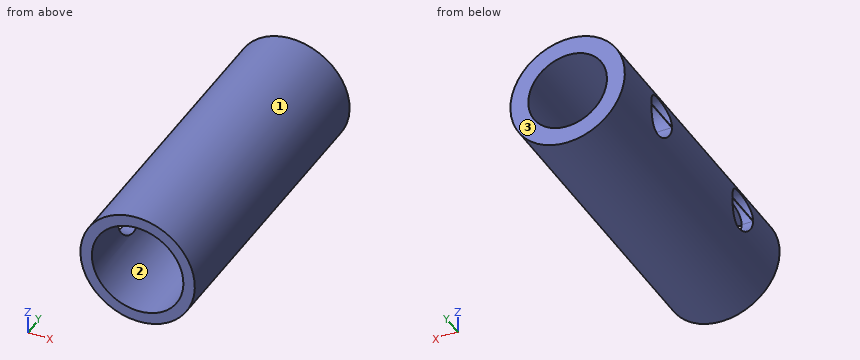
```python
from build123d import *

# Parameters (mm, degrees)
SKETCH1_R           = 4
BOSS_EXTRUDE1_DEPTH = 21
SKETCH2_R           = 3.2
CUT_EXTRUDE1_DEPTH  = 10
SKETCH3_R           = 2.75
CUT_EXTRUDE3_DEPTH  = 10


with BuildPart() as part:
    # Sketch1 → Boss-Extrude1 (new body)
    with BuildSketch(Plane(origin=(0, 0, 0), x_dir=(1, 0, 0), z_dir=(0, 1, 0))):
        with Locations(Location((0, 0, 0), (0, 0, 90))):
            Circle(SKETCH1_R)
    extrude(amount=BOSS_EXTRUDE1_DEPTH)

    # Sketch2 → Cut-Extrude1 (cut)
    with BuildSketch(Plane.XZ):
        with Locations(Location((0, 0, 0), (0, 0, 270))):
            Circle(SKETCH2_R)
    extrude(amount=-CUT_EXTRUDE1_DEPTH, mode=Mode.SUBTRACT)

    # Sketch3 → Cut-Extrude3 (cut)
    with BuildSketch(Plane(origin=(0, 21, 0), x_dir=(1, 0, 0), z_dir=(0, 1, 0))):
        with Locations(Location((0, 0, 0), (0, 0, 270))):
            Circle(SKETCH3_R)
    extrude(amount=-CUT_EXTRUDE3_DEPTH, mode=Mode.SUBTRACT)

    # Cut-Extrude5: read off the stored shape, not the designer's step
    # Cut-Extrude5: loft between two sections, ruled curve by curve
    cut_extrude5_from = [
        Edge.make_three_point_arc((-2.36677924, 14.6, 0), (-2.36677924, 16, 1.4), (-2.36677924, 17.4, 0)),
        Edge.make_three_point_arc((-2.36677924, 17.4, 0), (-2.36677924, 16, -1.4), (-2.36677924, 14.6, 0)),
    ]
    cut_extrude5_to = [
        Edge.make_three_point_arc((-3.999916451, 14.6, 0), (-3.999916451, 16, 1.4), (-3.999916451, 17.4, 0)),
        Edge.make_three_point_arc((-3.999916451, 17.4, 0), (-3.999916451, 16, -1.4), (-3.999916451, 14.6, 0)),
    ]
    cut_extrude5 = Solid(Shell([*[Face.make_surface_from_curves(cut_extrude5_from[k], cut_extrude5_to[k]) for k in range(2)], Face(Wire(cut_extrude5_from)), Face(Wire(cut_extrude5_to))]))
    add(cut_extrude5, mode=Mode.SUBTRACT)

    # Cut-Extrude5 2: loft between two sections, ruled curve by curve
    cut_extrude5_2_from = [
        Edge.make_three_point_arc((-2.877351837, 3.6, 0), (-2.877351837, 5, 1.4), (-2.877351837, 6.4, 0)),
        Edge.make_three_point_arc((-2.877351837, 6.4, 0), (-2.877351837, 5, -1.4), (-2.877351837, 3.6, 0)),
    ]
    cut_extrude5_2_to = [
        Edge.make_three_point_arc((-3.999916451, 3.6, 0), (-3.999916451, 5, 1.4), (-3.999916451, 6.4, 0)),
        Edge.make_three_point_arc((-3.999916451, 6.4, 0), (-3.999916451, 5, -1.4), (-3.999916451, 3.6, 0)),
    ]
    cut_extrude5_2 = Solid(Shell([*[Face.make_surface_from_curves(cut_extrude5_2_from[k], cut_extrude5_2_to[k]) for k in range(2)], Face(Wire(cut_extrude5_2_from)), Face(Wire(cut_extrude5_2_to))]))
    add(cut_extrude5_2, mode=Mode.SUBTRACT)


solid = part.part
```
Here's how the part is built. I have some questions about the finished solid (model axes, mm). Face numbers are marked on the shaded views. Round coordinates to 2 decimals unless told otherwise and drop trailing zeros. Order: outer loops, then holes, each group sorted by start corner. A loop starts at its lowest first (then second) coordinate and runs counter-clockwise, first axis right, second up. Notation, with made-up numbers: (28.5, 34.5) -> (41.5, 34.5) arc R16 cw to (41.5, 59.5) -> close; hole circle Ø10 at (24.5, 49). An arc over 180 degrees is marked (long way). Use a Markdown table: item, result. Add a question column.
(1) I need wall thicknesses on line 1 along X through (y, z) = (2.5, 0); line 2 along Y through (x, z) = (0.75, 1); line 3 along X through (y, z) = (15.75, 2.25). Which ranges of each line are inside material? Lowest first, please.
(2) Suppose I cut it at B-B, the plane y = 19. Please give me the cut outline in (x, z).
(3) Suppose I cut it at C-C, the plane z = -0.75. Count the separate pieces of the cut face and the enclosed holes in it, and give its area (3 significant figures).
(4) Suppose I cut it at D-D, the plane x = 2. Please give me the cut outline in (y, z).
(5) Suppose I cut it at A-A, the plane x = 0. Please give me the cut outline in (y, z).
(6) If we mould it in two halves opening along X, with no side actions, what happens to the marked faces 1, 2 and 3? For each: released by +X, released by -X, zero draft, split by the parting line, or undercut.
(7) For pin 1 Ø1 at (x, z) = (-2.5, -0.5) entering from +Y; pin 2 Ø3 at (x, z) = (1, 0.5) entering from +Y; pin 3 Ø1.9 at (x, z) = (-1, 0.5) entering from -Y; pin 4 Ø1 at (x, y) = (-2, 4.5) entering from +Z, each with a flat end and sliding along its axis, tell me the tip position at first contact or that it passes through.
Verdict:
| question | item | result |
|---|---|---|
| 1 | line 1 | -4 to -3.2, 3.2 to 4 |
| 1 | line 2 | 10 to 11 |
| 1 | line 3 | -3.31 to -1.58, 1.58 to 3.31 |
| 2 | outline | circle Ø8 at (0, 0); hole circle Ø5.5 at (0, 0) |
| 3 | separate pieces | 3 |
| 3 | enclosed holes | 0 |
| 3 | area | 44.9 mm2 |
| 4 | outline | (0, -3.46) -> (21, -3.46) -> (21, -1.89) -> (11, -1.89) -> (11, 1.89) -> (21, 1.89) -> (21, 3.46) -> (0, 3.46) -> (0, 2.5) -> (10, 2.5) -> (10, -2.5) -> (0, -2.5) -> close |
| 5 | outline | (0, -4) -> (21, -4) -> (21, -2.75) -> (11, -2.75) -> (11, 2.75) -> (21, 2.75) -> (21, 4) -> (0, 4) -> (0, 3.2) -> (10, 3.2) -> (10, -3.2) -> (0, -3.2) -> close |
| 6 | face 1 | split by the parting line |
| 6 | face 2 | undercut |
| 6 | face 3 | zero draft |
| 7 | pin 1 | y = 21 |
| 7 | pin 2 | y = 11 |
| 7 | pin 3 | y = 10 |
| 7 | pin 4 | z = 3.71 |
